Solid Edge part; units mm, degrees
sketch "Sketch1" plane through (0, 0, 0) normal (0, -1, 0) x (1, 0, 0)
  circle A0 centre (0, 0) radius 2
extrude "Protrusion1" add sketch "Sketch1" along normal blind 20.7
sketch "Sketch2" plane through (0, 0, 0) normal (0, 1, 0) x (1, 0, 0)
  line L0 (2.4942, -1.4332) -> (0, -2.8732)
  line L1 (-2.4942, -1.4332) -> (0, -2.8732)
  line L2 (-2.4942, 1.4468) -> (-2.4942, -1.4332)
  line L3 (0, 2.8868) -> (-2.4942, 1.4468)
  line L4 (0, 2.8868) -> (2.4942, 1.4468)
  line L5 (2.4942, 1.4468) -> (2.4942, -1.4332)
extrude "ExtrudedProtrusion_2" add sketch "Sketch2" along normal blind 2
fillet "Round_1" radius 0.2 12 edges at (1.2471, 0, 2.1532) (-1.2471, 0, 2.1532) (2.4942, 0, -0.0068) (1.2471, 0, -2.1668) (-1.2471, 0, -2.1668) (-2.4942, 0, -0.0068) (1.2471, 2, 2.1532) (-1.2471, 2, 2.1532) (-2.4942, 2, -0.0068) (-1.2471, 2, -2.1668) (1.2471, 2, -2.1668) (2.4942, 2, -0.0068)
fillet "Round_2" radius 0.2 18 edges at (0, 1, 2.8732) (0, 0.0586, 2.8056) (0, 1.9414, 2.8056) (2.4942, 1, 1.4332) (2.4356, 0.0586, 1.3994) (2.4356, 1.9414, 1.3994) (2.4942, 1, -1.4468) (2.4356, 0.0586, -1.4129) (2.4356, 1.9414, -1.4129) (-2.4942, 1, 1.4332) (-2.4356, 0.0586, 1.3994) (-2.4356, 1.9414, 1.3994) (0, 1, -2.8868) (0, 0.0586, -2.8191) (0, 1.9414, -2.8191) (-2.4942, 1, -1.4468) (-2.4356, 0.0586, -1.4129) (-2.4356, 1.9414, -1.4129)
chamfer "Chamfer_1" distance 0.5 angle 45 1 edges at (-2, -20.7, 0)
properties material "PVC"
Can you work these out from the model? Positions are in its coordinate system, mm. A direction names the side the tool comes from. Give positions to 0.01 mm unless a question says otherwise; leave off trailing zeros. Loops run counter-clockwise (first coordinate to the right, second up) from the corner with the lowest first, then second, coordinate; pieces in that order, holes last. Notation, with made-up numbers: (34.5, 80.25) -> (52.5, 80.25) arc R20 cw to (52.5, 116.25) -> close; hole circle Ø4 at (32, 81). An arc over 180 degrees is marked (long way). Write item = value, one per line.
1) Suppose I cut it at B-B on y = -1.5. Write out the boundary of the cut face in (x, z), then the cut area to 3 significant figures.
Check result:
outline = circle Ø4 at (0, 0)
area = 12.6 mm2
2) I need wall thicknesses on L1, parallel to Z at x = -0.1, y = -13.5; L2, parallel to Y at x = -2.1, z = 1.4; L3, parallel to Z at x = -1.4, y = -0.5. Which ranges of each line are inside material? Lowest first, please. Write a range as from..to.
Check result:
L1 = -2..2
L2 = 0..2
L3 = -1.43..1.43
3) Will this pin go through, and if not, where does the flat tip stop? pin 1 (1.5 mm diameter, centred on x = -1.5, y = -5.5, fed in from +Z).
Check result:
pin_1 = 1.85
4) For faces 1 (the flat face through (-1.231, 0.989, -2.176)), 2 (the cylindrical face through (0, -10, 2)), which set-ups out of +Z, -Z, +X, -X, +Y, -Y let a thin tool reach every point of the face, with its end or its side?
Check result:
face_1 = -Z, -X, +Y, -Y
face_2 = -Y
5) Suppose I cut it at A-A on z = 0. Write out the boundary of the cut face in (x, y).
Check result:
outline = (-2.49, 0.2) arc R0.2 ccw to (-2.29, 0) -> (-2, 0) -> (-2, -20.2) -> (-1.5, -20.7) -> (1.5, -20.7) -> (2, -20.2) -> (2, 0) -> (2.29, 0) arc R0.2 ccw to (2.49, 0.2) -> (2.49, 1.8) arc R0.2 ccw to (2.29, 2) -> (-2.29, 2) arc R0.2 ccw to (-2.49, 1.8) -> close
